from build123d import *

# Parameters (mm, degrees)
SKETCH1_W           = 20
SKETCH1_H           = 12
BOSS_EXTRUDE1_DEPTH = 26
SKETCH2_W           = 10
SKETCH2_H           = 12
BOSS_EXTRUDE2_DEPTH = 8
SKETCH4_R           = 1.55
CUT_EXTRUDE2_DEPTH  = 41.049968789
FILLET1_R           = 3
FILLET3_R           = 3
SKETCH5_W           = 9.976745634
SKETCH5_H           = 0.5
SKETCH5_W_2         = 12.25993895
CUT_EXTRUDE3_DEPTH  = 41.049968789
SKETCH6_W           = 5.5
SKETCH6_H           = 30.488056323
CUT_EXTRUDE4_DEPTH  = 0.8
SKETCH8_W           = 12
SKETCH8_H           = 12
BOSS_EXTRUDE3_DEPTH = 40
SKETCH3_R           = 1.8
CUT_EXTRUDE1_DEPTH  = 73.691127382
SKETCH9_R           = 1.5
CUT_EXTRUDE6_DEPTH  = 12
FILLET4_R           = 4
SKETCH10_R          = 1.45
CUT_EXTRUDE7_DEPTH  = 12
FILLET5_R           = 4
FILLET7_R           = 4


with BuildPart() as part:
    # Sketch1 → Boss-Extrude1 (new body)
    with BuildSketch(Plane.XY):
        with Locations((10, -6)):
            Rectangle(SKETCH1_W, SKETCH1_H)
    extrude(amount=BOSS_EXTRUDE1_DEPTH)

    # Sketch2 → Boss-Extrude2 (add)
    with BuildSketch(Plane(origin=(20, 0, 0), x_dir=(0, 0, -1), z_dir=(1, 0, 0))):
        with Locations((-21, -6)):
            Rectangle(SKETCH2_W, SKETCH2_H)
    extrude(amount=BOSS_EXTRUDE2_DEPTH)

    # Sketch4 → Cut-Extrude2 (cut, through all)
    with BuildSketch(Plane(origin=(0, 0, 0), x_dir=(1, 0, 0), z_dir=(0, 1, 0))):
        with Locations(Location((13, -15.5, 0), (0, 0, 270))):
            Circle(SKETCH4_R)
        with Locations(Location((6, -15.5, 0), (0, 0, 270))):
            Circle(SKETCH4_R)
    extrude(amount=-CUT_EXTRUDE2_DEPTH, mode=Mode.SUBTRACT)

    # Fillet1
    fillet1_edges = [part.edges().sort_by_distance(p)[0] for p in [
        (20, -6, 16),
    ]]
    fillet(fillet1_edges, radius=FILLET1_R)

    # Fillet3
    fillet3_edges = [part.edges().sort_by_distance(p)[0] for p in [
        (10, 0, 0),
        (10, -12, 0),
    ]]
    fillet(fillet3_edges, radius=FILLET3_R)

    # Sketch5 → Cut-Extrude3 (cut, through all)
    with BuildSketch(Plane.ZY):
        with Locations((0.011627183, -11.75)):
            Rectangle(SKETCH5_W, SKETCH5_H)
        with Locations((-1.129969475, -0.25)):
            Rectangle(SKETCH5_W_2, SKETCH5_H)
    extrude(amount=-CUT_EXTRUDE3_DEPTH, mode=Mode.SUBTRACT)

    # Sketch6 → Cut-Extrude4 (cut)
    with BuildSketch(Plane(origin=(0, 0, 0), x_dir=(-1, 0, 0), z_dir=(0, 0, -1))):
        with Locations((-10, -7.868232937)):
            Rectangle(SKETCH6_W, SKETCH6_H)
    extrude(amount=-CUT_EXTRUDE4_DEPTH, mode=Mode.SUBTRACT)

    # Sketch8 → Boss-Extrude3 (add)
    with BuildSketch(Plane.XY.offset(26)):
        with Locations((22, -6)):
            Rectangle(SKETCH8_W, SKETCH8_H)
    extrude(amount=BOSS_EXTRUDE3_DEPTH)

    # Sketch3 → Cut-Extrude1 (cut, through all)
    with BuildSketch(Plane.ZY):
        with Locations(Location((5, -6, 0), (0, 0, 270))):
            Circle(SKETCH3_R)
    extrude(amount=-CUT_EXTRUDE1_DEPTH, mode=Mode.SUBTRACT)

    # Sketch9 → Cut-Extrude6 (cut)
    with BuildSketch(Plane(origin=(28, 0, 0), x_dir=(0, 0, -1), z_dir=(1, 0, 0))):
        with Locations((-31, -6)):
            Circle(SKETCH9_R)
        with Locations((-38, -6)):
            Circle(SKETCH9_R)
        with Locations((-45, -6)):
            Circle(SKETCH9_R)
        with Locations((-52, -6)):
            Circle(SKETCH9_R)
        with Locations((-59, -6)):
            Circle(SKETCH9_R)
    extrude(amount=-CUT_EXTRUDE6_DEPTH, mode=Mode.SUBTRACT)

    # Fillet4
    fillet4_edges = [part.edges().sort_by_distance(p)[0] for p in [
        (16, -6, 26),
    ]]
    fillet(fillet4_edges, radius=FILLET4_R)

    # Sketch10 → Cut-Extrude7 (cut)
    with BuildSketch(Plane.XY.offset(26)):
        with Locations((8, -6)):
            Circle(SKETCH10_R)
    extrude(amount=-CUT_EXTRUDE7_DEPTH, mode=Mode.SUBTRACT)

    # Fillet5
    fillet5_edges = [part.edges().sort_by_distance(p)[0] for p in [
        (28, -6, 16),
    ]]
    fillet(fillet5_edges, radius=FILLET5_R)

    # Fillet7
    fillet7_edges = [part.edges().sort_by_distance(p)[0] for p in [
        (22, 0, 66),
        (22, -12, 66),
    ]]
    fillet(fillet7_edges, radius=FILLET7_R)


solid = part.part
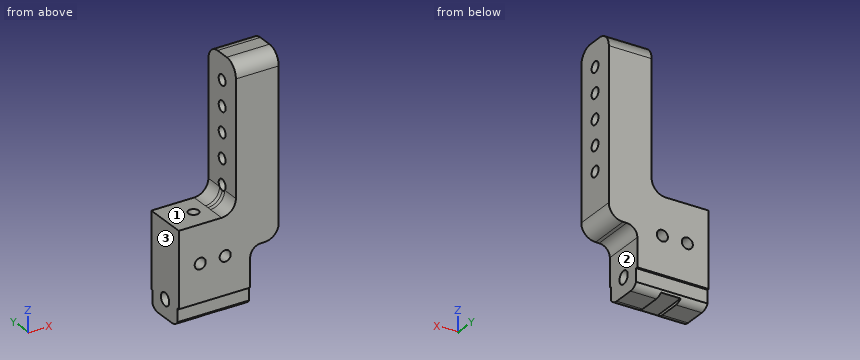
CAD build for the part. Positions are in the model's coordinates, mm. Face numbers are marked on the shaded views. A direction names the side the tool comes from. Give positions to 0.01 mm unless a question says otherwise; leave off trailing zeros. Write each loop counter-clockwise with the first axis right and the second up, starting at its lowest first coordinate (ties: lowest second). Pieces come first, ordered by that corner, then holes. Notation, with made-up numbers: (-16.75, 49) -> (22.25, 49) arc R26 ccw to (22.25, 72) -> close; hole circle Ø5 at (-39.5, 18.5). An arc over 180 degrees is marked (long way). Return JSON: item names as keys, results as strings.
Item 1: Band-saw the part on D-D (z = 54.5). List the corners of the cut face in (x, y), then the cut area to 3 significant figures.
Answer below:
{"outline": "(16, -12) -> (28, -12) -> (28, 0) -> (16, 0) -> close", "area": "144 mm2"}
Item 2: Band-saw the part on C-C (y = -10.25). List the corners of the cut face in (x, z).
Answer below:
{"outline": "(0, 0.27) -> (7.25, 0.27) -> (7.25, 0.8) -> (12.75, 0.8) -> (12.75, 0.27) -> (20, 0.27) -> (20, 13) arc R3 cw to (23, 16) -> (24, 16) arc R4 ccw to (28, 20) -> (28, 65.31) -> (16, 65.31) -> (16, 30) arc R4 cw to (12, 26) -> (0, 26) -> close; hole circle Ø3.1 at (6, 15.5); hole circle Ø3.1 at (13, 15.5)"}
Item 3: Band-saw the part on A-A (x = 18.25). List the corners of the cut face in (y, z).
Answer below:
{"outline": "(-12, 5) -> (-11.5, 5) -> (-11.5, 1.34) arc R3 ccw to (-9, 0) -> (-3, 0) arc R3 ccw to (-0.5, 1.34) -> (-0.5, 5) -> (0, 5) -> (0, 62) arc R4 ccw to (-4, 66) -> (-8, 66) arc R4 ccw to (-12, 62) -> close; hole circle Ø3.6 at (-6, 5); hole circle Ø3 at (-6, 31); hole circle Ø3 at (-6, 38); hole circle Ø3 at (-6, 45); hole circle Ø3 at (-6, 52); hole circle Ø3 at (-6, 59)"}
Item 4: Drop flat-ended pins along their axis: pin 1 (0.9 mm diameter, centred on x = 8, y = -6.5, fed in from +Z); pin 2 (8 mm diameter, centred on x = 13.5, z = 57.5, fed in from -Y); pin 3 (3.5 mm diameter, centred on y = -7.5, z = 3.5, fed in from +X); pin 4 (3.5 mm diameter, centred on y = -5, z = 56, fed in from -X). Give the stop position or say it passes through.
Answer below:
{"pin 1": "stops at z = 14", "pin 2": "stops at y = -12", "pin 3": "stops at x = 20", "pin 4": "stops at x = 16"}
Item 5: Band-saw the part on B-B (z = 45). List the corners of the cut face in (x, y), then the cut area to 3 significant figures.
Answer below:
{"outline": "(16, -12) -> (28, -12) -> (28, -7.5) -> (16, -7.5) -> close; (16, -4.5) -> (28, -4.5) -> (28, 0) -> (16, 0) -> close", "area": "108 mm2"}
Item 6: Drill centre lines: probe 1 along Y at (x, z) = (22, 31); probe 2 along Y at (x, z) = (8, 20.5); probe 3 along Z at (x, y) = (7, -4.75). Where is each one in solid material? Low to high.
Answer below:
{"probe 1": "y = -12 to -7.5, -4.5 to 0", "probe 2": "y = -12 to -7.45, -4.55 to 0", "probe 3": "z = 0 to 3.7, 6.3 to 14.32, 16.68 to 26"}
Item 7: Tool access for the marked faces 1, 2 and 3: list every direction of +Z, -Z, +X, -X, +Y, -Y with a clear straight run to the whole face (end or side of a thin tool).
Answer below:
{"face 1": "+Z, -X, +Y, -Y", "face 2": "-Z, +X, +Y, -Y", "face 3": "+Z, -Z, -X, +Y, -Y"}
